Design review of the part built by this model. Coordinates are the model's own, in mm. Face numbers are marked on the shaded views. Coordinates: 2 decimals unless noted, no trailing zeros. Write each loop counter-clockwise with the first axis right and the second up, starting at its lowest first coordinate (ties: lowest second). Pieces come first, ordered by that corner, then holes. Notation, with made-up numbers: M 18,-39.75 L 59,-39.75 A34 cw 59,-2.75 Z; hole C 81,15 d7. An arc over 180 degrees is marked long. One line per question, with ' | ' between items.
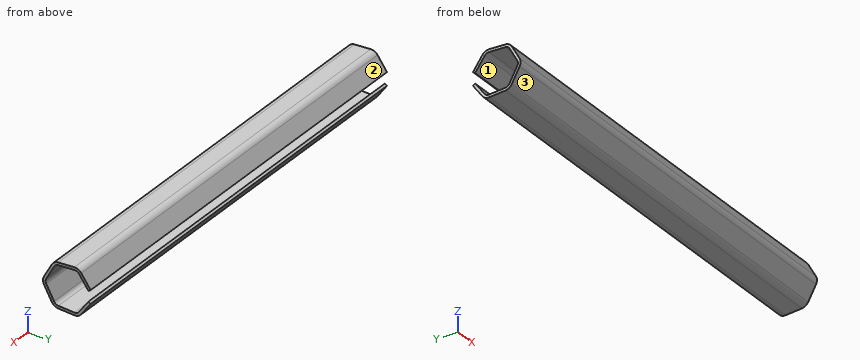
from build123d import *

# Parameters (mm, degrees)
EXTRUDE_THIN1_DEPTH = 325


with BuildPart() as part:
    # Sketch1 → Extrude-Thin1 (new, symmetric)
    with BuildSketch(Plane(origin=(0, 0, 0), x_dir=(0, 0, -1), z_dir=(1, 0, 0))):
        with BuildLine():
            Line((10, 36.492499074), (30.033921668, 22.128857106))
            ThreePointArc((30.033921668, 22.128857106), (33.873815741, 17.540413964), (35.020847295, 11.668198405))
            Line((35.020847295, 11.668198405), (33.565953275, -12.939839131))
            ThreePointArc((33.565953275, -12.939839131), (31.734968696, -18.635986288), (27.381153255, -22.739995068))
            Line((27.381153255, -22.739995068), (5.79428183, -34.642902698))
            ThreePointArc((5.79428183, -34.642902698), (0, -36.134510905), (-5.79428183, -34.642902698))
            Line((-5.79428183, -34.642902698), (-27.381153255, -22.739995068))
            ThreePointArc((-27.381153255, -22.739995068), (-31.734968696, -18.635986288), (-33.565953275, -12.939839131))
            Line((-33.565953275, -12.939839131), (-35.020847295, 11.668198405))
            ThreePointArc((-35.020847295, 11.668198405), (-33.873815741, 17.540413964), (-30.033921668, 22.128857106))
            Line((-30.033921668, 22.128857106), (-10, 36.492499074))
            Line((-10, 36.492499074), (-7.669281259, 33.241691459))
            Line((-7.669281259, 33.241691459), (-27.703202927, 18.878049491))
            ThreePointArc((-27.703202927, 18.878049491), (-30.263132309, 15.819087397), (-31.027820011, 11.904277024))
            Line((-31.027820011, 11.904277024), (-29.572925992, -12.703760512))
            ThreePointArc((-29.572925992, -12.703760512), (-28.352269606, -16.50119195), (-25.449725978, -19.237197803))
            Line((-25.449725978, -19.237197803), (-3.862854553, -31.140105433))
            ThreePointArc((-3.862854553, -31.140105433), (0, -32.134510905), (3.862854553, -31.140105433))
            Line((3.862854553, -31.140105433), (25.449725978, -19.237197803))
            ThreePointArc((25.449725978, -19.237197803), (28.352269606, -16.50119195), (29.572925992, -12.703760512))
            Line((29.572925992, -12.703760512), (31.027820011, 11.904277024))
            ThreePointArc((31.027820011, 11.904277024), (30.263132309, 15.819087397), (27.703202927, 18.878049491))
            Line((27.703202927, 18.878049491), (7.669281259, 33.241691459))
            Line((7.669281259, 33.241691459), (10, 36.492499074))
        make_face()
    extrude(amount=EXTRUDE_THIN1_DEPTH, both=True)


solid = part.part
1. Take a section at B-B (z = -19). Write out the cut boundary in (x, y).
Answer sheet:
outline: M -325,-27.36 L 325,-27.36 L 325,-22.79 L -325,-22.79 Z; M -325,25.12 L 325,25.12 L 325,30.04 L -325,30.04 Z
2. Insertion check: pin 1 Ø2 at (x, z) = (-153.5, -11.5) entering from +Y; pin 2 Ø8 at (x, y) = (199.5, -12.5) entering from +Z; pin 3 Ø10 at (x, z) = (113.5, -22) entering from +Y. Each pin has a flat end and moves straight along its axis. Give the tip position at first contact, or say it passes through.
Answer sheet:
pin 1: y = 36.13 | pin 2: z = 33.83 | pin 3: y = 31.47
3. To check wall thickness, follow line 1 along Z through (x, y) = (264, 12); line 2 along Z through (x, y) = (-177.5, -13); line 3 along Y through (x, z) = (205.5, -10.5). State the ranges of each line that lie inside material, in increasing order. Write a range as [from, to].
Answer sheet:
line 1: [-35.04, -31.03], [31.03, 35.04] | line 2: [-33.56, -29.55], [29.55, 33.56] | line 3: [-32.05, -27.48], [31.21, 36.13]
4. Take a section at C-C (x = 75). Write out the cut boundary in (y, z).
Answer sheet:
outline: M -34.64,-5.79 L -22.74,-27.38 A12 ccw -12.94,-33.57 L 11.67,-35.02 A12 ccw 22.13,-30.03 L 36.49,-10 L 33.24,-7.67 L 18.88,-27.7 A8 cw 11.9,-31.03 L -12.7,-29.57 A8 cw -19.24,-25.45 L -31.14,-3.86 A8 cw -31.14,3.86 L -19.24,25.45 A8 cw -12.7,29.57 L 11.9,31.03 A8 cw 18.88,27.7 L 33.24,7.67 L 36.49,10 L 22.13,30.03 A12 ccw 11.67,35.02 L -12.94,33.57 A12 ccw -22.74,27.38 L -34.64,5.79 A12 ccw Z
5. Draft analysis for pull direction Z (two halves, no side actions). For the marked faces 1, 2 and 3, state which applies: pulls with the +Z half, pulls with the -Z half, needs draft (parallel to the pull), parting line crosses it, or undercut.
Answer sheet:
face 1: undercut | face 2: pulls with the +Z half | face 3: pulls with the -Z half
6. Take a section at A-A (y = 1). Write out the cut boundary in (x, z), then the cut area to 3 significant figures.
Answer sheet:
outline: M -325,-34.39 L 325,-34.39 L 325,-30.38 L -325,-30.38 Z; M -325,30.38 L 325,30.38 L 325,34.39 L -325,34.39 Z | area: 5,210 mm^2
